For this review, take the finished solid that the model builds, in its own axes (mm). A direction names the side the tool comes from. Round coordinates to 2 decimals unless told otherwise and drop trailing zeros. Write each loop counter-clockwise with the first axis right and the second up, starting at its lowest first coordinate (ties: lowest second). Pieces come first, ordered by that corner, then holes. Notation, with made-up numbers: (-31.5, -19.5) -> (27.5, -19.5) arc R10 cw to (27.5, -3.5) -> close; hole circle Ø8 at (58.5, 60.5). An arc over 180 degrees is marked (long way). Write each question's results on one line, items separated by ' | '. Start each with the question number.
Item 1: Clearance check with a flat-ended pin moving along its axis: pin 1 (4.5 mm diameter, centred on y = 41, z = 0, fed in from -X). State where the tip first meets the part, or that it passes through.
Item 2: The part is to be moulded in two halves that separate along X. For faces 1 (the flat face through (-7.5, 158, 0)), 2 (the flat face through (-6.5, 158, 0)), 3 (the flat face through (-7, 0, 0)), say which applies: +X half, -X half, draft (parallel to the pull), parting line (faces both ways), or undercut.
Item 3: To check wall thickness, follow line 1 along Y through (x, z) = (-7.1, 0); line 2 along Z through (x, y) = (-2.5, 116.5). State the ranges of each line that lie inside material, in increasing order.
Item 4: Add section B-B (y = 52.5). State the section outline as (x, z) points.
Item 5: Add section C-C (z = 4.25). State the section outline as (x, y) points.
Item 6: Add section A-A (x = 4.25). State the section outline as (y, z) points.
Item 7: Tool access review of faces 4 (the flat face through (7.5, 158, 0)), 5 (the flat face through (6.5, 158, 0)): name each direction out of +Z, -Z, +X, -X, +Y, -Y from which nothing blocks a thin tool from reaching the whole face with its end or side.
from build123d import *

# Parameters (mm, degrees)
SKETCH_1_W          = 15
SKETCH_1_H          = 15
SKETCH_1_W_2        = 13
SKETCH_1_H_2        = 13
EXTRUDE_1_DEPTH     = 320
SKETCH_3_R          = 2
CUT_EXTRUDE_2_DEPTH = 321.43915179
SKETCH_4_R          = 2
CUT_EXTRUDE_3_DEPTH = 321.43915179


with BuildPart() as part:
    # 草图1 → 凸台-拉伸1 (new body)
    with BuildSketch(Plane(origin=(0, 0, 0), x_dir=(1, 0, 0), z_dir=(0, 1, 0))):
        Rectangle(SKETCH_1_W, SKETCH_1_H)
        Rectangle(SKETCH_1_W_2, SKETCH_1_H_2, mode=Mode.SUBTRACT)
    extrude(amount=EXTRUDE_1_DEPTH)

    # 草图3 → 切除-拉伸2 (cut, through all)
    with BuildSketch(Plane.XY.offset(7.5)):
        with Locations((0, 295)):
            Circle(SKETCH_3_R)
        with Locations((0, 275)):
            Circle(SKETCH_3_R)
        with Locations(Location((0, 45, 0), (0, 0, 180))):
            Circle(SKETCH_3_R)
        with Locations(Location((0, 25, 0), (0, 0, 180))):
            Circle(SKETCH_3_R)
        with Locations((0, 255)):
            Circle(SKETCH_3_R)
        with Locations(Location((0, 65, 0), (0, 0, 180))):
            Circle(SKETCH_3_R)
    extrude(amount=-CUT_EXTRUDE_2_DEPTH, mode=Mode.SUBTRACT)

    # 草图4 → 切除-拉伸3 (cut, through all)
    with BuildSketch(Plane.ZY.offset(7.5)):
        with Locations((0, 11)):
            Circle(SKETCH_4_R)
        with Locations((0, 41)):
            Circle(SKETCH_4_R)
        with Locations(Location((0, 279, 0), (0, 0, 180))):
            Circle(SKETCH_4_R)
        with Locations(Location((0, 309, 0), (0, 0, 180))):
            Circle(SKETCH_4_R)
    extrude(amount=-CUT_EXTRUDE_3_DEPTH, mode=Mode.SUBTRACT)


solid = part.part
Responses:
1) pin 1: stops at x = -7.5
2) face 1: -X half | face 2: undercut | face 3: draft
3) line 1: y = 0 to 9, 13 to 39, 43 to 277, 281 to 307, 311 to 320 | line 2: z = -7.5 to -6.5, 6.5 to 7.5
4) outline: (-7.5, -7.5) -> (7.5, -7.5) -> (7.5, 7.5) -> (-7.5, 7.5) -> close; hole (-6.5, -6.5) -> (6.5, -6.5) -> (6.5, 6.5) -> (-6.5, 6.5) -> close
5) outline: (-7.5, 0) -> (-6.5, 0) -> (-6.5, 320) -> (-7.5, 320) -> close; (6.5, 0) -> (7.5, 0) -> (7.5, 320) -> (6.5, 320) -> close
6) outline: (0, -7.5) -> (320, -7.5) -> (320, -6.5) -> (0, -6.5) -> close; (0, 6.5) -> (320, 6.5) -> (320, 7.5) -> (0, 7.5) -> close
7) face 4: +Z, -Z, +X, +Y, -Y | face 5: +Y, -Y
